Study the drawing (mm; zero at the part's minimum x, y, z) and answer. A direction names the side the tool comes from. Round coordinates to 2 decimals unless told otherwise and drop trailing zeros. Order: outer loops, then holes, each group sorted by start corner. A loop starts at its lowest first (then second) coordinate and runs counter-clockwise, first axis right, second up. Notation, with made-up numbers: (13.25, -23) - (28.25, -23) arc R27 ccw to (28.25, 4) - close; hole circle Ø7 at (-2, 74.25). An arc over 180 degrees is marked (long way). Use one line per item in the form item = value. Start each with the question number.
Q1. The part is cut by section D-D on z = 32. Determine the outline of the cut face in (x, y).
Q2. Which of the six approach directions +Z, -Z, +X, -X, +Y, -Y give full straight-line access (tool end or side, diameter ignored) to the marked faces 5 and 6?
Q3. Given P1, Ø8, axis at x = 5.5, z = 43.5, coming from the -Y side (1 decimal); P2, Ø10, axis at x = 12.5, z = 44.5, coming from the +Y side; P3, Ø7, axis at x = 15, z = 10.5, coming from the +Y side, each flat-ended and moving along its own axis, determine where each tip first touches the part or whether it passes through.
Q4. Find the intervals of material crossed by line 1 (Y direction, x = 18, z = 15); line 2 (Z direction, x = 6, y = 14); line 3 (Z direction, x = 9.5, y = 2.5), in increasing order. Write a range as [from, to].
Q5. The part is cut by section C-C on y = 4. Determine the outline of the cut face in (x, z).
Q6. The part is cut by section A-A on z = 20.5. Determine the outline of the cut face in (x, y).
Q7. For a pull along Y with two mould halves and no side action, classify the marked faces 1, 2, 3 and 4 as +Y half, -Y half, draft (parallel to the pull), parting line (faces both ways), or undercut.
Q8. The part is cut by section B-B on x = 22.5. Determine the outline of the cut face in (y, z), plus the area to 3 significant figures.
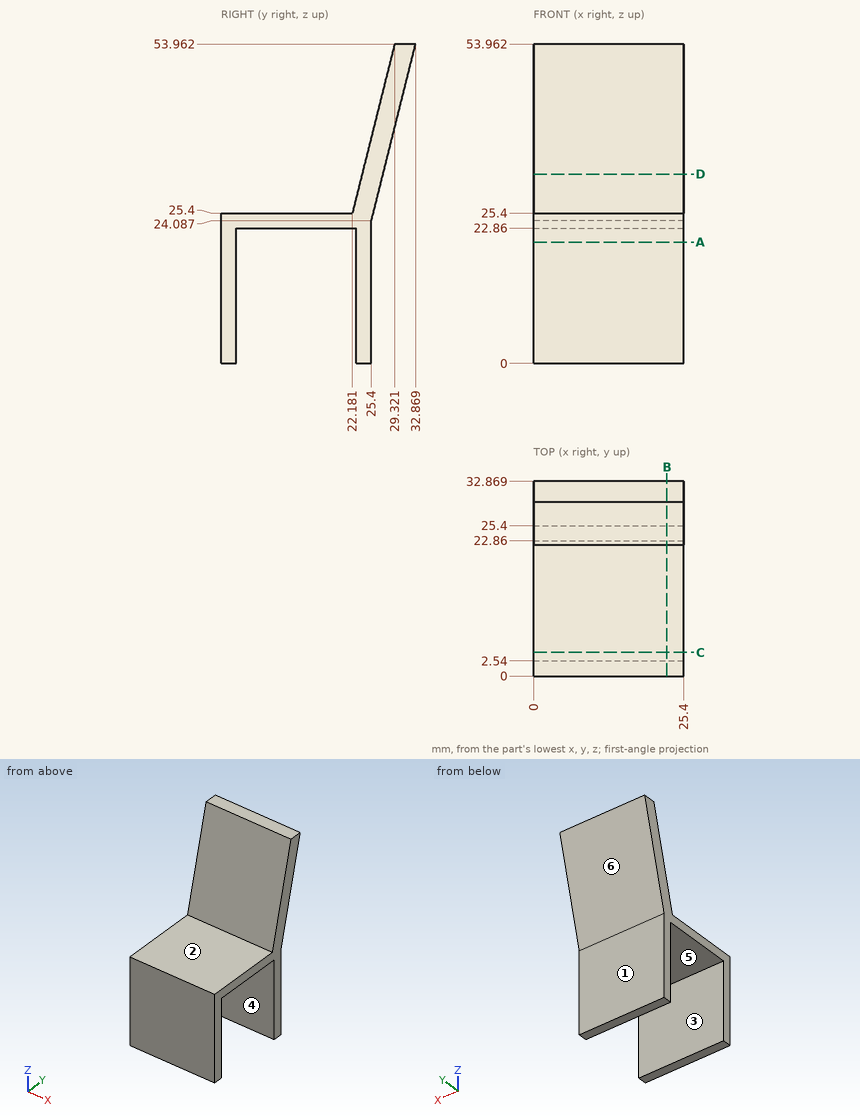
Found:
q1.outline = (0, 23.83) - (25.4, 23.83) - (25.4, 27.38) - (0, 27.38) - close
q2.face_5 = -Z, +X, -X
q2.face_6 = -Z, +X, -X, +Y
q3.P1 = 25.7
q3.P2 = 31.75
q3.P3 = 25.4
q4.line_1 = [0, 2.54], [22.86, 25.4]
q4.line_2 = [22.86, 25.4]
q4.line_3 = [0, 25.4]
q5.outline = (0, 22.86) - (25.4, 22.86) - (25.4, 25.4) - (0, 25.4) - close
q6.outline = (0, 0) - (25.4, 0) - (25.4, 2.54) - (0, 2.54) - close; (0, 22.86) - (25.4, 22.86) - (25.4, 25.4) - (0, 25.4) - close
q7.face_1 = +Y half
q7.face_2 = draft
q7.face_3 = undercut
q7.face_4 = undercut
q8.outline = (0, 0) - (2.54, 0) - (2.54, 22.86) - (22.86, 22.86) - (22.86, 0) - (25.4, 0) - (25.4, 24.09) - (32.87, 53.96) - (29.32, 53.96) - (22.18, 25.4) - (0, 25.4) - close
q8.area = 282 mm²
